Answer from the drawing. Dimensions are ordinates in mm from the lowest x, y and z of the part. Coordinates: 2 decimals unless noted, no trailing zeros. Order: outer loops, then holes, each group sorted by start corner. A loop starts at its lowest first (then second) coordinate and runs counter-clockwise, first axis right, second up. Notation, with made-up numbers: (5.25, 61.5) - (18.25, 61.5) arc R10 ccw to (18.25, 77.5) - close; hole circle Ø1 at (58, 11). An arc over 180 degrees is marked (long way). Answer as a JSON object with one key per item and string values. Group by question number.
1) Section B-B (z = 0.55) is taken. Count the separate pieces of the cut face and the enclosed holes in it, plus the area to 3 significant figures.
2) Section C-C (x = 16) is taken. Give the vertices of the cut face in (y, z), plus the area to 3 significant figures.
3) Each of these flat-tipped pins is pushed along its axis until it touches: P1, Ø0.8, axis at x = 14, z = 2, coming from the -Y side; P2, Ø1.5, axis at x = 18.5, z = 2, coming from the +Y side; P3, Ø1.5, axis at y = 53, z = 1, coming from the +X side. Where does it stop, or does it pass through?
4) Find the intervals of material crossed by line 1 along X through (y, z) = (41.5, 1.5); line 2 along Y through (x, z) = (5.5, 0.65); line 3 along X through (y, z) = (49, 0.4), in increasing order.
5) Section A-A (y = 14) is taken. Give the vertices of the cut face in (x, z).
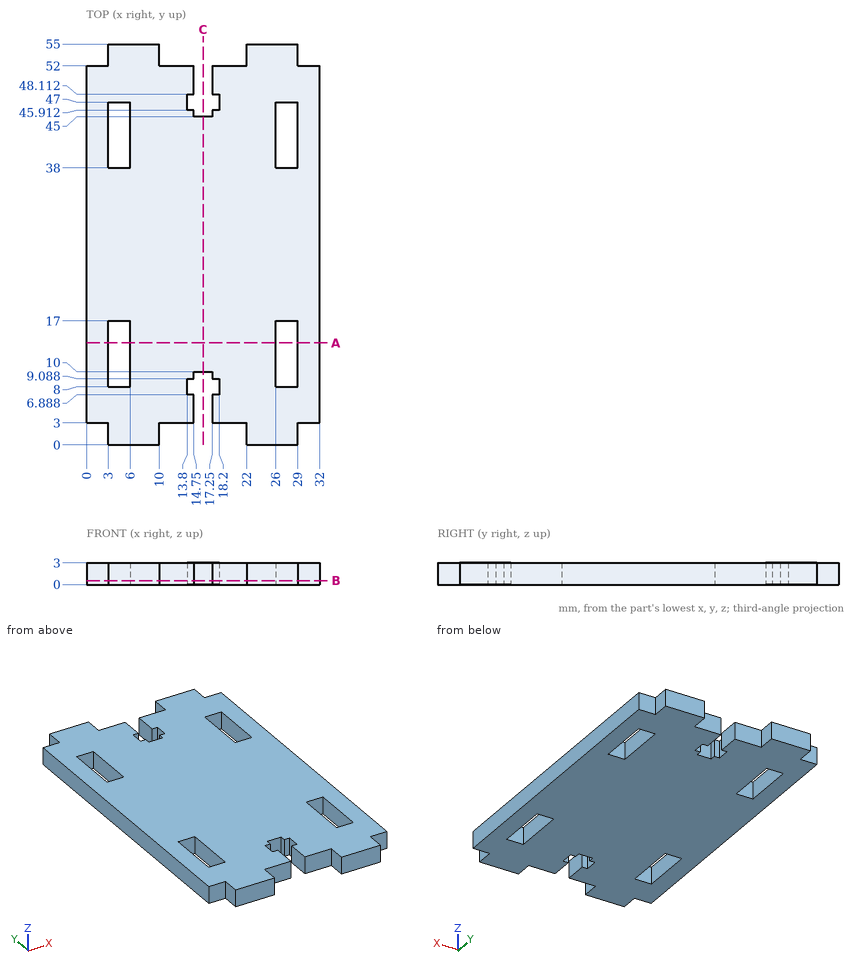
Report:
{
 "1": {"separate pieces": "1", "enclosed holes": "4", "area": "1,500 mm²"},
 "2": {"outline": "(10, 0) - (45, 0) - (45, 3) - (10, 3) - close", "area": "105 mm²"},
 "3": {"P1": "stops at y = 3", "P2": "stops at y = 52", "P3": "stops at x = 29"},
 "4": {"line 1": "x = 0 to 3, 6 to 26, 29 to 32", "line 2": "y = 0 to 8, 17 to 38, 47 to 55", "line 3": "x = 0 to 14.75, 17.25 to 32"},
 "5": {"outline": "(0, 0) - (3, 0) - (3, 3) - (0, 3) - close; (6, 0) - (26, 0) - (26, 3) - (6, 3) - close; (29, 0) - (32, 0) - (32, 3) - (29, 3) - close"}
}
